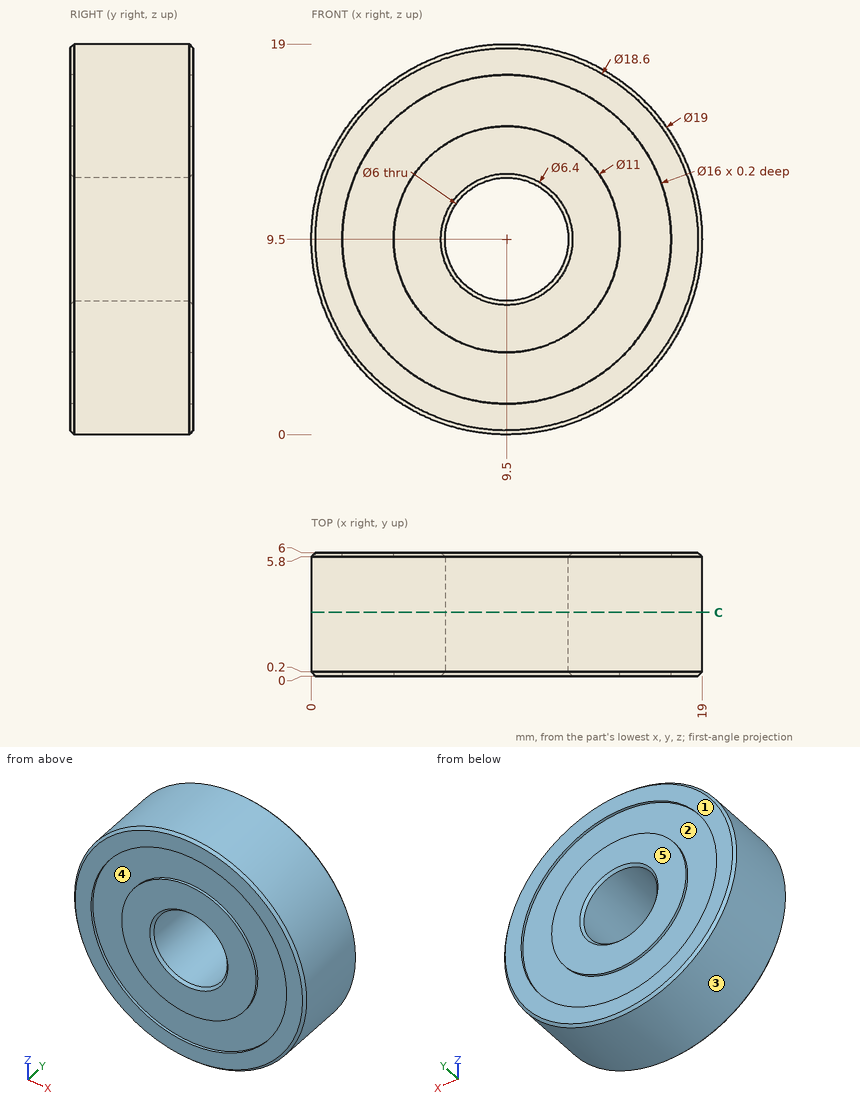
Source: three-view drawing plus pictorial views. Frame: mm from the lowest corner of the part. A direction names the side the tool comes from. Give positions to 0.01 mm unless a question says otherwise; leave off trailing zeros. Write each loop counter-clockwise with the first axis right and the second up, starting at its lowest first coordinate (ties: lowest second). Pieces come first, ordered by that corner, then holes.
(1) Cut plane C-C, the plane y = 3.1. Return loops of the section in (x, z).
(2) Access query for the marked faces 4 and 5. Directions: +Z, -Z, +X, -X, +Y, -Y. A direction counts if a zero-diameter tool reaches every point of the face in a straight line with its end or side. Return the directions, or none.
(3) First-contact query: P1, Ø2, axis at x = 4, y = 1, coming from the -Z side; P2, Ø3, axis at x = 14.5, y = 3, coming from the +Z side; P3, Ø1.5, axis at x = 16, y = 2, coming from the +Z side; P4, Ø5, axis at x = 9.5, z = 9.5, coming from the -Y side. Flat tips, straight axial feed; report the tip coordinate or a pass-through.
(4) Mould query, pull axis X, two halves, no side actions, for the marked faces 1, 2 and 3. Classes: released by +X, released by -X, zero draft, split by the parting line, or undercut.
(5) Ray query, line 1 (X direction, y = 5.9, z = 9.5); line 2 (Z direction, x = 9.5, y = 2.95); line 3 (Z direction, x = 9.5, y = 5.95). Return the intervals inside material, ascending.
Values follow:
1. outline: circle Ø19 at (9.5, 9.5); hole circle Ø6 at (9.5, 9.5)
2. face 4: -Y
2. face 5: +Z, -Z, +X, -X, +Y
3. P1: stops at z = 1.13
3. P2: stops at z = 18.33
3. P3: stops at z = 17.06
3. P4: passes through
4. face 1: zero draft
4. face 2: undercut
4. face 3: split by the parting line
5. line 1: x = 0.1 to 1.5, 4 to 6.4, 12.6 to 15, 17.5 to 18.9
5. line 2: z = 0 to 6.5, 12.5 to 19
5. line 3: z = 0.15 to 1.5, 4 to 6.35, 12.65 to 15, 17.5 to 18.85
